The listing builds one solid part. Answer for the finished solid, in the listing's coordinates (mm). A direction names the side the tool comes from. Round coordinates to 2 decimals unless told otherwise and drop trailing zeros. Write each loop counter-clockwise with the first axis right and the second up, starting at its lowest first coordinate (ties: lowest second). Pieces come first, ordered by that corner, then holes.
Item 1: Find the intervals of material crossed by probe 1 along Y at (x, z) = (7.4, 3.4); probe 2 along Y at (x, z) = (12.7, 4.05); probe 3 along Y at (x, z) = (18.5, 1.5), in increasing order.
Item 2: Each of these flat-tipped pins is pushed along its axis until it touches: pin 1 (5 mm diameter, centred on x = -4.5, y = -52, fed in from +Z); pin 2 (5.5 mm diameter, centred on x = 18.4, y = 4, fed in from +Z); pin 3 (1.5 mm diameter, centred on y = -66, z = 8, fed in from +X); pin 4 (6 mm diameter, centred on x = -1, z = 10, fed in from +Y). Where does it stop, or does it pass through?
Item 3: Find section D-D on y = -23. Give the vertices of the cut face in (x, z).
Item 4: A tool of negligible diameter and unlimited length cuts with its end or side. For faces 4 (the face through (24.648, 24.287, 3.035)), 5 (the face through (-8.341, -46.068, 3.117)), from which of +Z, -Z, +X, -X, +Y, -Y can it reach the whole face along a straight path? Write none if from no direction.
Item 5: Find section B-B on y = -42.7. Give the vertices of the cut face in (x, z).
Item 6: For a pull along X with two mould halves and no side action, classify faces 1 (the face through (-25.4, -30, 3)), 2 (the face through (-7, -54, 0.8)), 3 (the face through (24.393, -83.026, 5.865)) as +X half, -X half, draft (parallel to the pull), parting line (faces both ways), or undercut.
Item 7: Find section A-A on x = 12.7. Give the number of separate pieces and of enclosed holes in the cut face, then the cut area to 3 significant figures.
```python
from build123d import *

# Parameters (mm, degrees)
MAIN_FEATURES_SKETCH_W         = 50.8
MAIN_FEATURES_SKETCH_H         = 109
MAIN_FEATURES_SKETCH_R         = 3.4925
MAIN_FEATURES_SKETCH_R_2       = 8
MAIN_BODY_DEPTH                = 6
SKETCH1_5_W                    = 45.8
SKETCH1_5_H                    = 5
LEDGE_DEPTH                    = 12
SKETCH1_4_R                    = 8
SCREW_HEAD_RECESSES_DEPTH      = 0.8
M5X0_8_TAPPED_HOLE1_AT_2_COUNT = 2
M5X0_8_TAPPED_HOLE1_AT_2_PITCH = 25
M5X0_8_TAPPED_HOLE1_AT_3_COUNT = 2
M5X0_8_TAPPED_HOLE1_AT_3_PITCH = 16.650825805
FILLET1_R                      = 2.5
CHAMFER1_SIZE                  = 0.5


with BuildPart() as part:
    # main_features_sketch → main_body (new body)
    with BuildSketch(Plane.XY):
        with Locations((0, -29.5)):
            Rectangle(MAIN_FEATURES_SKETCH_W, MAIN_FEATURES_SKETCH_H)
        with Locations((12.7, -42.7)):
            Circle(MAIN_FEATURES_SKETCH_R, mode=Mode.SUBTRACT)
        with Locations((12.7, -68.1)):
            Circle(MAIN_FEATURES_SKETCH_R, mode=Mode.SUBTRACT)
        with Locations((-7.3, -54)):
            Circle(MAIN_FEATURES_SKETCH_R_2, mode=Mode.SUBTRACT)
        with Locations((-7.3, -74)):
            Circle(MAIN_FEATURES_SKETCH_R_2, mode=Mode.SUBTRACT)
        with Locations((-12.7, -42.7)):
            Circle(MAIN_FEATURES_SKETCH_R, mode=Mode.SUBTRACT)
    extrude(amount=MAIN_BODY_DEPTH)

    # Sketch1<5> → ledge (add)
    with BuildSketch(Plane.XY):
        with Locations((0, -27.5)):
            Rectangle(SKETCH1_5_W, SKETCH1_5_H)
    extrude(amount=LEDGE_DEPTH)

    # Sketch1<4> → screw_head_recesses (add)
    with BuildSketch(Plane.XY):
        with Locations((-7.3, -54)):
            Circle(SKETCH1_4_R)
        with Locations((-7.3, -74)):
            Circle(SKETCH1_4_R)
    extrude(amount=SCREW_HEAD_RECESSES_DEPTH)

    # Sketch3 → M5x0.8 Tapped Hole1 (revolve, cut)
    with BuildSketch(Plane(origin=(7.4, -8.5, 6), x_dir=(0, -1, 0), z_dir=(1, 0, 0))):
        Polygon((0, 0), (0, 6), (2.525, 6), (2.1, 5.575), (2.1, 0.425), (2.525, 0), align=None)
    m5x0_8_tapped_hole1 = revolve(axis=Axis((7.4, -8.5, 12.35), (0, 0, -1)), mode=Mode.SUBTRACT)

    # M5x0.8 Tapped Hole1 at 2: M5x0.8 Tapped Hole1 ×2
    with Locations(*[(0, i * M5X0_8_TAPPED_HOLE1_AT_2_PITCH, 0) for i in range(1, M5X0_8_TAPPED_HOLE1_AT_2_COUNT)]):
        add(m5x0_8_tapped_hole1, mode=Mode.SUBTRACT)

    # M5x0.8 Tapped Hole1 at 3: M5x0.8 Tapped Hole1 ×2
    with Locations(*[Vector(0.6606278948920246, 0.7507135169227555, 0) * (i * M5X0_8_TAPPED_HOLE1_AT_3_PITCH) for i in range(1, M5X0_8_TAPPED_HOLE1_AT_3_COUNT)]):
        add(m5x0_8_tapped_hole1, mode=Mode.SUBTRACT)

    # Fillet1
    fillet1_edges = [part.edges().sort_by_distance(p)[0] for p in [
        (25.4, 25, 3),
        (-25.4, 25, 3),
        (25.4, -84, 3),
        (-25.4, -84, 3),
        (22.9, -25, 9),
        (22.9, -30, 9),
        (-22.9, -25, 9),
        (-22.9, -30, 9),
    ]]
    fillet(fillet1_edges, radius=FILLET1_R - 0.0001)  # a hair under: the kernel refuses the full size

    # Chamfer1
    chamfer1_edges = [part.edges().sort_by_distance(p)[0] for p in [
        (0, 25, 0),
        (-24.667796242, 24.267796242, 0),
        (24.667796242, 24.267796242, 0),
        (-24.667796242, -83.267796242, 0),
        (24.667796242, -83.267796242, 0),
        (0, -84, 6),
        (0, 25, 6),
        (-25.4, -29.5, 6),
        (-24.667796242, 24.267796242, 6),
        (24.667796242, 24.267796242, 6),
        (-24.667796242, -83.267796242, 6),
        (24.667796242, -83.267796242, 6),
        (-16.1925, -42.7, 0),
        (9.2075, -42.7, 0),
        (9.2075, -68.1, 0),
        (9.2075, -68.1, 6),
        (-15.3, -74, 6),
        (-15.3, -54, 6),
        (9.2075, -42.7, 6),
        (-16.1925, -42.7, 6),
        (0, -25, 12),
        (0, -30, 12),
        (-22.167796242, -29.267796242, 12),
        (-22.167796242, -25.732203758, 12),
        (22.167796242, -29.267796242, 12),
        (22.167796242, -25.732203758, 12),
        (25.4, -29.5, 0),
        (25.4, -29.5, 6),
        (0, -84, 0),
        (-25.4, -29.5, 0),
    ]]
    chamfer(chamfer1_edges, length=CHAMFER1_SIZE)


solid = part.part
```
Check values:
1. probe 1: y = -84 to -10.6, -6.4 to 14.4, 18.6 to 25
1. probe 2: y = -84 to -71.59, -64.61 to -46.19, -39.21 to 25
1. probe 3: y = -84 to 1.9, 6.1 to 25
2. pin 1: stops at z = 0.8
2. pin 2: stops at z = 6
2. pin 3: passes through
2. pin 4: stops at y = -25
3. outline: (-25.4, 0.5) - (-24.9, 0) - (24.9, 0) - (25.4, 0.5) - (25.4, 5.5) - (24.9, 6) - (-24.9, 6) - (-25.4, 5.5) - close
4. face 4: +Z, -Z, +X, +Y
4. face 5: +Z
5. outline: (-25.4, 0.5) - (-24.9, 0) - (-16.69, 0) - (-16.19, 0.5) - (-16.19, 5.5) - (-16.69, 6) - (-24.9, 6) - (-25.4, 5.5) - close; (-9.21, 0.5) - (-8.71, 0) - (8.71, 0) - (9.21, 0.5) - (9.21, 5.5) - (8.71, 6) - (-8.71, 6) - (-9.21, 5.5) - close; (16.19, 0.5) - (16.69, 0) - (24.9, 0) - (25.4, 0.5) - (25.4, 5.5) - (24.9, 6) - (16.69, 6) - (16.19, 5.5) - close
6. face 1: -X half
6. face 2: undercut
6. face 3: +X half
7. separate pieces: 3
7. enclosed holes: 0
7. area: 598 mm2
